For this review, take the finished solid that the model builds, in its own axes (mm). A direction names the side the tool comes from. Give positions to 0.01 mm unless a question says otherwise; leave off trailing zeros. Write each loop counter-clockwise with the first axis right and the second up, starting at its lowest first coordinate (ties: lowest second). Pieces come first, ordered by that corner, then holes. Notation, with made-up numbers: M 14,-27.75 L 71,-27.75 A16 ccw 71,-4.75 Z; hole C 84,-21 d2. An arc over 180 degrees is marked long. One line per item, written item: value. Start each with the question number.
Item 1: Consider section A-A, the plane z = 26. Write out the cut boundary in (x, y), and give its area (3 significant figures).
Item 2: To check wall thickness, follow probe 1 along Y at (x, z) = (-0.5, 24); probe 2 along X at (y, z) = (5.25, 37); probe 3 along Z at (x, y) = (-8, 4.5). State the ranges of each line that lie inside material, in increasing order.
Item 3: Consider section D-D, the plane x = -30. Write out the cut boundary in (y, z).
Item 4: Consider section B-B, the plane x = 8.5. Write out the cut boundary in (y, z).
Item 5: Clearance check with flat-ended pins moving along their axes: pin 1 Ø19.5 at (x, z) = (22.5, 27) entering from -Y; pin 2 Ø5 at (x, y) = (3.5, 4) entering from -Z; pin 3 Ø0.6 at (y, z) = (5.5, 25) entering from +X; pin 4 Ø10 at (x, z) = (-40.5, 21) entering from -Y. State where each tip first meets the part, or that it passes through.
Item 6: Tool access review of faces 1 (the face through (61.4, 5.3, 3.06)), 2 (the face through (-61.4, 5.31, 3.06)), 3 (the face through (-1, 2, 42)), 4 (the face through (1, 5, 2.2)): name each direction out of +Z, -Z, +X, -X, +Y, -Y from which nothing blocks a thin tool from reaching the whole face with its end or side.
Item 7: Consider section C-C, the plane y = -1.5. Write out the cut boundary in (x, z).
Item 8: Mouldability with a two-part tool opening along Y and no side actions: class faces 5 (the face through (-1, 2.406, 20)), 6 (the face through (-1, 0, 0)), 7 (the face through (1, 4.206, 22)), 8 (the face through (-1, 5.906, 22)) as released by +Y, released by -Y, zero draft, split by the parting line, or undercut.
Solid Edge part; units mm, degrees
sketch "Sketch1" plane through (0, 0, 0) normal (0, 0, 1) x (1, 0, 0)
  arc A0 (-64, 1.9062) -> (64, 1.9062) centre (0, 295) ccw
  line L0 (64, 1.9062) -> (64, 5.9062)
  line L1 (-64, 5.9062) -> (64, 5.9062)
  line L2 (-64, 1.9062) -> (-64, 5.9062)
extrude "Protrusion1" add sketch "Sketch1" along normal blind 41.5
fillet "Verrundung_1" radius 3 1 edges at (-64, 3.9062, 0)
fillet "Verrundung_2" radius 3 1 edges at (64, 3.9062, 0)
sketch "Sketch2" plane through (0, -1.119, 41.5) normal (0, 0, 1) x (1, 0, 0)
  line L0 (-62.3, 7.0251) -> (-62.3, 5.8251)
  line L1 (-62.3, 5.8251) -> (-64, 5.8251)
  line L2 (-64, 5.8251) -> (-64, 7.0251)
  line L3 (-64, 7.0251) -> (-62.3, 7.0251)
  line L4 (64, 7.0251) -> (64, 5.8251)
  line L5 (64, 5.8251) -> (62.3, 5.8251)
  line L6 (62.3, 5.8251) -> (62.3, 7.0251)
  line L7 (62.3, 7.0251) -> (64, 7.0251)
extrude "Extrusionsausschnitt_1" cut sketch "Sketch2" against normal blind 45
sketch "Sketch3" plane through (0, 0.4531, 0) normal (0, 0, -1) x (1, 0, 0)
  line L0 (-61.5, -1.9531) -> (61.5, -1.9531)
  line L1 (61.5, -1.9531) -> (61.5, -3.7531)
  line L2 (61.5, -3.7531) -> (-61.5, -3.7531)
  line L3 (-61.5, -3.7531) -> (-61.5, -1.9531)
extrude "Extrusionsausschnitt_2" cut sketch "Sketch3" against normal blind 554.4
sketch "Sketch4" plane through (-62.3, 5.3062, 21.6481) normal (-1, 0, 0) x (0, 0, 1)
  line L0 (-21.6481, 0.6) -> (-19.4481, 0.6)
  line L1 (-19.4481, 0.6) -> (-19.4481, -2.9)
  line L2 (-21.6481, -2.9) -> (-19.4481, -2.9)
  line L3 (-21.6481, 0.6) -> (-21.6481, -2.9)
extrude "Extrusionsausschnitt_3" cut sketch "Sketch4" along normal blind 28.8 and the other way blind 145.8
fillet "Verrundung_3" radius 3 2 edges at (-62.3, 5.3062, 2.2) (62.3, 5.3062, 2.2)
sketch "Sketch5" plane through (0, 0.4531, 41.5) normal (0, 0, 1) x (1, 0, 0)
  line L0 (62.3, 5.4531) -> (-62.3, 5.4531)
  line L1 (-62.3, 5.4531) -> (-62.3, 4.2531)
  line L2 (-62.3, 4.2531) -> (-64, 4.2531)
  line L3 (-64, 4.2531) -> (-64, 1.4531)
  arc A0 (-64, 1.4531) -> (64, 1.4531) centre (0, 294.5469) ccw
  line L4 (64, 1.4531) -> (64, 4.2531)
  line L5 (64, 4.2531) -> (62.3, 4.2531)
  line L6 (62.3, 4.2531) -> (62.3, 5.4531)
extrude "Extrusionsausprägung_2" add sketch "Sketch5" along normal blind 0.5
Model answer:
1. outline: M -64,1.91 A300 ccw 64,1.91 L 64,4.71 L 62.3,4.71 L 62.3,5.91 L -62.3,5.91 L -62.3,4.71 L -64,4.71 Z; hole M -61.5,2.41 L 61.5,2.41 L 61.5,4.21 L -61.5,4.21 Z
1. area: 877 mm2
2. probe 1: y = -5 to 2.41, 4.21 to 5.91
2. probe 2: x = -62.3 to 62.3
2. probe 3: z = 2.2 to 42
3. outline: M -3.5,0 L 2.41,0 L 2.41,41.5 L 4.21,41.5 L 4.21,2.2 L 5.91,2.2 L 5.91,42 L -3.5,42 Z
4. outline: M -4.88,0 L 2.41,0 L 2.41,41.5 L 4.21,41.5 L 4.21,2.2 L 5.91,2.2 L 5.91,42 L -4.88,42 Z
5. pin 1: stops at y = -4.73
5. pin 2: stops at z = 0
5. pin 3: stops at x = 62.3
5. pin 4: stops at y = -2.89
6. face 1: -Z, +X, +Y
6. face 2: -Z, -X, +Y
6. face 3: +Z, +X, -X, +Y, -Y
6. face 4: -Z, +X, -X, +Y
7. outline: M -45.69,0 L 45.69,0 L 45.69,42 L -45.69,42 Z
8. face 5: undercut
8. face 6: zero draft
8. face 7: undercut
8. face 8: released by +Y
